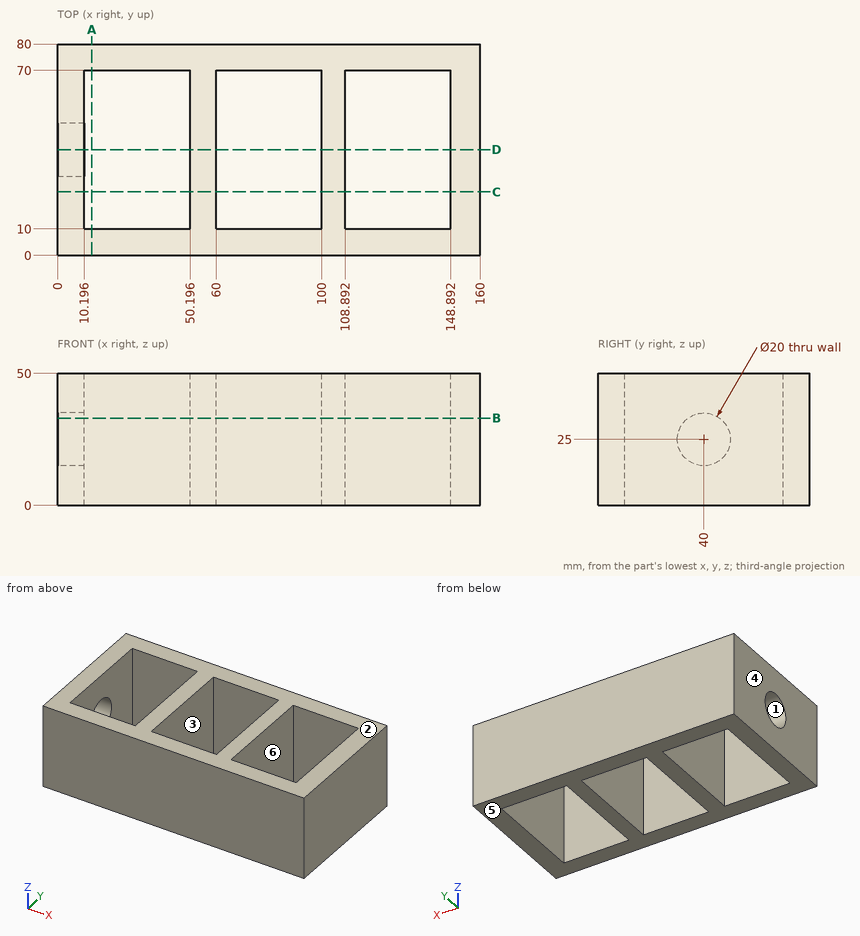
The figure shows three views and two pictorial views of one solid part (mm, origin at its lowest corner). Answer the questions. A direction names the side the tool comes from. Round coordinates to 2 decimals unless told otherwise and drop trailing zeros. Write each loop counter-clockwise with the first axis right and the second up, starting at its lowest first coordinate (ties: lowest second). Pieces come first, ordered by that corner, then holes. Notation, with made-up numbers: (56.5, 84) - (88.5, 84) arc R23 cw to (88.5, 117) - close; hole circle Ø5 at (80.5, 44). An arc over 180 degrees is marked (long way). One line per question, with ' | ' between items. Start each with the question number.
1. Find the intervals of material crossed by probe 1 along X at (y, z) = (53.5, 47.5); probe 2 along Y at (x, z) = (93, 32); probe 3 along Z at (x, y) = (7.75, 40), in increasing order. Write a range as [from, to].
2. Section C-C (y = 24) is taken. Determine the outline of the cut face in (x, z), and give its area (3 significant figures).
3. Section B-B (z = 33) is taken. Determine the outline of the cut face in (x, y).
4. Section D-D (y = 40) is taken. Determine the outline of the cut face in (x, z), and give its area (3 significant figures).
5. For the marked faces 1, 2 and 3, determine the directions among +Z, -Z, +X, -X, +Y, -Y from which every point of the face is accessible in a straight line to the end or side of a thin tool.
6. For a pull along X with two mould halves and no side action, classify the marked faces 4, 5 and 6 as +X half, -X half, draft (parallel to the pull), parting line (faces both ways), or undercut.
7. Section A-A (x = 13) is taken. Determine the outline of the cut face in (y, z).
8. This flat-tipped pin is pushed along its axis until it touches: pin 1 (18 mm diameter, centred on y = 40, z = 25, fed in from -X). Where does it stop, or does it pass through?
Filled in:
1) probe 1: [0, 10.2], [50.2, 60], [100, 108.89], [148.89, 160] | probe 2: [0, 10], [70, 80] | probe 3: [0, 15], [35, 50]
2) outline: (0, 0) - (10.2, 0) - (10.2, 50) - (0, 50) - close; (50.2, 0) - (60, 0) - (60, 50) - (50.2, 50) - close; (100, 0) - (108.89, 0) - (108.89, 50) - (100, 50) - close; (148.89, 0) - (160, 0) - (160, 50) - (148.89, 50) - close | area: 2,000 mm²
3) outline: (0, 0) - (160, 0) - (160, 80) - (0, 80) - (0, 46) - (10.2, 46) - (10.2, 70) - (50.2, 70) - (50.2, 10) - (10.2, 10) - (10.2, 34) - (0, 34) - close; hole (60, 10) - (100, 10) - (100, 70) - (60, 70) - close; hole (108.89, 10) - (148.89, 10) - (148.89, 70) - (108.89, 70) - close
4) outline: (0, 0) - (10.2, 0) - (10.2, 15) - (0, 15) - close; (0, 35) - (10.2, 35) - (10.2, 50) - (0, 50) - close; (50.2, 0) - (60, 0) - (60, 50) - (50.2, 50) - close; (100, 0) - (108.89, 0) - (108.89, 50) - (100, 50) - close; (148.89, 0) - (160, 0) - (160, 50) - (148.89, 50) - close | area: 1,800 mm²
5) face 1: -X | face 2: +Z, +X, -X, +Y, -Y | face 3: +Z, -Z
6) face 4: -X half | face 5: draft | face 6: undercut
7) outline: (0, 0) - (10, 0) - (10, 50) - (0, 50) - close; (70, 0) - (80, 0) - (80, 50) - (70, 50) - close
8) pin 1: x = 50.2
